```python
from build123d import *

# Parameters (mm, degrees)
FILLET1_R                  = 6
F_12_0_12_DIAMETER_HOLE1_D = 12
CIRPATTERN1_COUNT          = 4


with BuildPart() as part:
    # Sketch1 → Revolve1 (revolve)
    with BuildSketch(Plane.XY, mode=Mode.PRIVATE) as revolve1_sk:
        Polygon((0, 19), (0, 70), (20, 70), (20, 35), (50, 35), (50, 19), align=None)
    revolve(revolve1_sk.sketch.rotate(Axis((0, 0, 0), (1, 0, 0)), 90), axis=Axis((0, 0, 0), (1, 0, 0)))

    # Fillet1
    fillet1_edges = [part.edges().sort_by_distance(p)[0] for p in [
        (50, 0, -35),
        (20, 0, -35),
        (20, 0, -70),
    ]]
    fillet(fillet1_edges, radius=FILLET1_R)

    # Ø12.0 (12) Diameter Hole1 (through all)
    with Locations(Plane.ZY):
        with Locations((0, 55)):
            f_12_0_12_diameter_hole1 = Hole(F_12_0_12_DIAMETER_HOLE1_D / 2)

    # CirPattern1: Ø12.0 (12) Diameter Hole1 ×4 about axis
    cirpattern1_axis = Axis((0, 0, 0), (1, 0, 0))
    for i in range(1, CIRPATTERN1_COUNT):
        add(f_12_0_12_diameter_hole1.rotate(cirpattern1_axis, i * 360 / CIRPATTERN1_COUNT), mode=Mode.SUBTRACT)


solid = part.part
```
Input: part model. Units: mm. Frame: model coordinates. A direction names the side the tool comes from. Give positions to 0.01 mm unless a question says otherwise; leave off trailing zeros. Order: outer loops, then holes, each group sorted by start corner. A loop starts at its lowest first (then second) coordinate and runs counter-clockwise, first axis right, second up.
1. Mould query, pull axis Z, two halves, no side actions, for faces 3 (the flat face through (0, 15, -15)), 4 (the cylindrical face through (10.14, 1.301, -49.143)), 5 (the cylindrical face through (10.14, -49.143, -1.301)), 6 (the cylindrical face through (7.098, 68.335, -15.175)). Classes: released by +Z, released by -Z, zero draft, split by the parting line, or undercut.
Derived:
face 3: zero draft
face 4: undercut
face 5: undercut
face 6: split by the parting line
2. Reachability of faces 1 (the cylindrical face through (10.14, 49.143, 1.301)), 2 (the flat face through (20, 42, -1)) from +Z, -Z, +X, -X, +Y, -Y: full face, straight path, thin tool, end or side. Return the list, or none.
Derived:
face 1: +X, -X
face 2: +X
3. Section C-C on x = 16. Return the cut outline in (y, z), and give its area (3 significant figures).
Derived:
outline: circle Ø139.31 at (0, 0); hole circle Ø12 at (-55, 0); hole circle Ø38 at (0, 0); hole circle Ø12 at (0, -55); hole circle Ø12 at (0, 55); hole circle Ø12 at (55, 0)
area: 13,700 mm2
4. Section A-A on y = 0. Return the cut outline in (x, z).
Derived:
outline: (0, -70) - (14, -70) arc R6 ccw to (20, -64) - (20, -61) - (0, -61) - close; (0, -49) - (20, -49) - (20, -41) arc R6 cw to (26, -35) - (44, -35) arc R6 ccw to (50, -29) - (50, -19) - (0, -19) - close; (0, 19) - (50, 19) - (50, 29) arc R6 ccw to (44, 35) - (26, 35) arc R6 cw to (20, 41) - (20, 49) - (0, 49) - close; (0, 61) - (20, 61) - (20, 64) arc R6 ccw to (14, 70) - (0, 70) - close
5. Pin query (flat end, axial travel): pin 1 (9.5 mm diameter, centred on y = 55, z = 0, fed in from -X); pin 2 (6 mm diameter, centred on x = 35.5, y = -16.5, fed in from -Z); pin 3 (6 mm diameter, centred on x = 37, y = -32.5, fed in from +Z); pin 4 (4 mm diameter, centred on x = 10.5, z = 10.5, fed in from +Y). Return the tip coordinate at first contact, or that it passes through.
Derived:
pin 1: passes through
pin 2: stops at z = -32.29
pin 3: stops at z = 18.83
pin 4: stops at y = 69.48
6. Section B-B on x = 36. Return the cut outline in (y, z), and give its area (3 significant figures).
Derived:
outline: circle Ø70 at (0, 0); hole circle Ø38 at (0, 0)
area: 2,710 mm2
7. Material intervals for L1, parallel to Y at x = 8, z = 0; L2, parallel to Y at x = 30, z = 0; L3, parallel to Y at x = 16, z = 0, sorted ascending.
Derived:
L1: y = -70 to -61, -49 to -19, 19 to 49, 61 to 70
L2: y = -35 to -19, 19 to 35
L3: y = -69.66 to -61, -49 to -19, 19 to 49, 61 to 69.66
